Design review of the part shown in the three views and the two pictorial views. Dimensions are in mm from the part's minimum x, y and z. A direction names the side the tool comes from. Coordinates: 2 decimals unless noted, no trailing zeros. Loops run counter-clockwise (first coordinate to the right, second up) from the corner with the lowest first, then second, coordinate; pieces in that order, holes last.
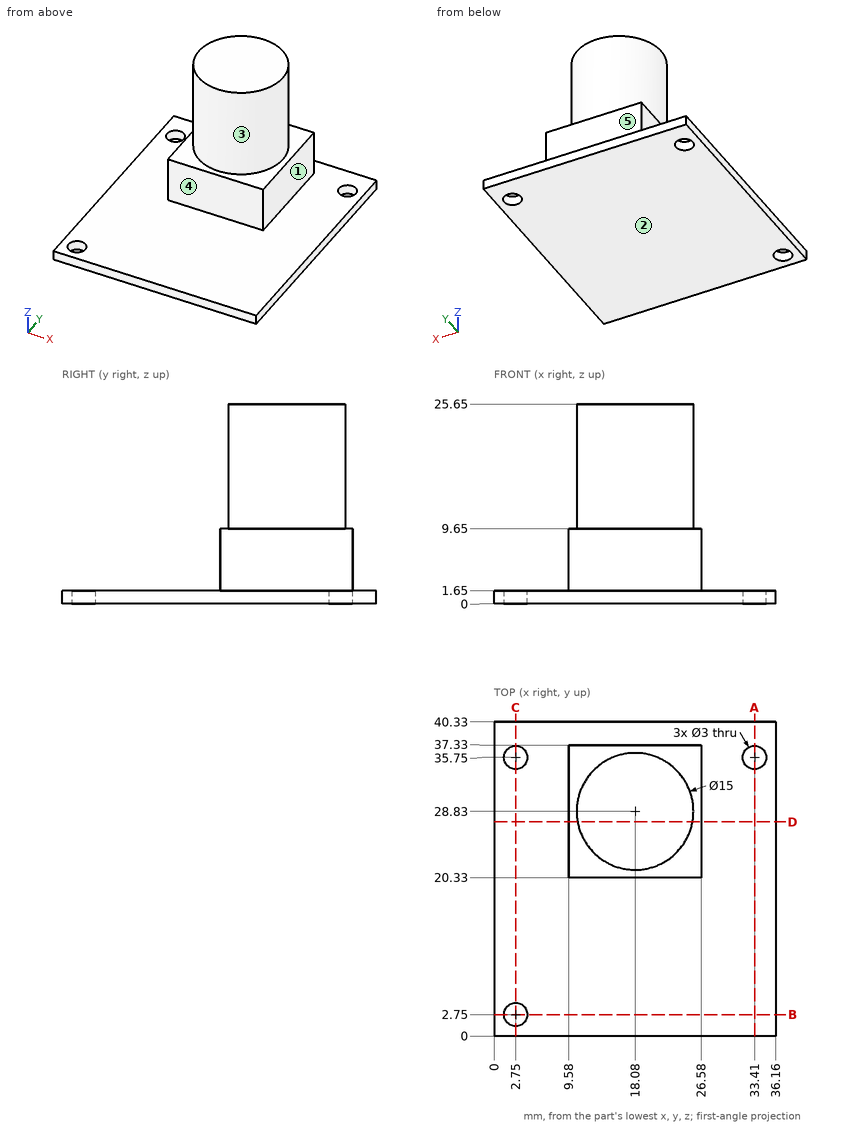
Q1. Consider section A-A (x = 33.41). State the section outline as (y, z) points.
Q2. Consider section B-B (y = 2.75). State the section outline as (x, z) points.
Q3. Machinability: for the marked faces 1, 2, 3, 4 and 5, which of the approach directions +Z, -Z, +X, -X, +Y, -Y give a long, thin tool a straight path to every point of the face, cutting with its end or side? Answer none if there is none.
Q4. Wall thickness on probe 1 along Y at (x, z) = (2.75, 0.45); probe 2 along X at (y, z) = (35.75, 0.5); probe 3 along X at (y, z) = (2.75, 1.05): over which ranges is each line inside the solid? List them lowest first.
Q5. Consider section D-D (y = 27.5). State the section outline as (x, z) points, then the cut area to 3 significant figures.
Q6. For pin 1 Ø10 at (x, z) = (6.5, 10.5) entering from +Y; pin 2 Ø2.5 at (x, y) = (2.75, 2.75) entering from -Z; pin 3 Ø6.5 at (x, z) = (16.5, 6) entering from -Y; pin 4 Ø5 at (x, y) = (33.41, 35.75) entering from +Z, all flat-tipped, find the tip position at first contact; note any pin that passes through.
Q7. Consider section C-C (x = 2.75). State the section outline as (y, z) points.
Model answer:
1. outline: (0, 0) - (34.25, 0) - (34.25, 1.65) - (0, 1.65) - close; (37.25, 0) - (40.33, 0) - (40.33, 1.65) - (37.25, 1.65) - close
2. outline: (0, 0) - (1.25, 0) - (1.25, 1.65) - (0, 1.65) - close; (4.25, 0) - (36.16, 0) - (36.16, 1.65) - (4.25, 1.65) - close
3. face 1: +Z, +X, +Y, -Y
3. face 2: -Z, +X, -X, +Y, -Y
3. face 3: +Z
3. face 4: +Z, +X, -X, -Y
3. face 5: +Z, +X, -X, +Y
4. probe 1: y = 0 to 1.25, 4.25 to 34.25, 37.25 to 40.33
4. probe 2: x = 0 to 1.25, 4.25 to 31.91, 34.91 to 36.16
4. probe 3: x = 0 to 1.25, 4.25 to 36.16
5. outline: (0, 0) - (36.16, 0) - (36.16, 1.65) - (26.58, 1.65) - (26.58, 9.65) - (25.46, 9.65) - (25.46, 25.65) - (10.7, 25.65) - (10.7, 9.65) - (9.58, 9.65) - (9.58, 1.65) - (0, 1.65) - close
5. area: 432 mm2
6. pin 1: stops at y = 37.33
6. pin 2: passes through
6. pin 3: stops at y = 20.33
6. pin 4: stops at z = 1.65
7. outline: (0, 0) - (1.25, 0) - (1.25, 1.65) - (0, 1.65) - close; (4.25, 0) - (34.25, 0) - (34.25, 1.65) - (4.25, 1.65) - close; (37.25, 0) - (40.33, 0) - (40.33, 1.65) - (37.25, 1.65) - close
